```python
from build123d import *

# Parameters (mm, degrees)
F0_R      = 6.35
F1_DEPTH  = 47.625
F3_DEPTH  = 31.75
F4_R      = 23.8125
F4_R_2    = 18.7325
F5_DEPTH  = 20.32
F6_R      = 54.61
F6_R_2    = 6.35
F7_DEPTH  = 14.605
F8_R      = 54.5973
F8_R_2    = 6.35
F9_DEPTH  = 118.491
F10_R     = 54.61
F10_R_2   = 54.5973
F10_R_3   = 6.35
F11_DEPTH = 57.15
F13_DEPTH = 101.6
F15_DEPTH = 25.4
F16_DEPTH = 76.2
F18_DEPTH = 76.2
F20_D     = 12.7
F20_DEPTH = 12.7
F20_TIP   = 3.8154649308
F22_D     = 12.7
F22_2_D   = 12.7
F23_R     = 5.08
F23_2_R   = 5.08


with BuildPart() as f1:
    # F0 (on Top) → F1 (new body)
    with BuildSketch(Plane.XY):
        Circle(F0_R)
    extrude(amount=-F1_DEPTH)

    # F2 (on face) → F3 (cut)
    with BuildSketch(Plane.XY):
        with BuildLine():
            Line((-3.4925, 5.3032955556), (3.4925, 5.3032955556))
            ThreePointArc((3.4925, 5.3032955556), (0, 6.35), (-3.4925, 5.3032955556))
        make_face()
    extrude(amount=-F3_DEPTH, mode=Mode.SUBTRACT)


with BuildPart() as f5:
    # F4 (on face) → F5 (new body)
    with BuildSketch(Plane(origin=(0, 0, -47.625), x_dir=(1, 0, 0), z_dir=(0, 0, -1))):
        Circle(F4_R)
        Circle(F4_R_2, mode=Mode.SUBTRACT)
    extrude(amount=-F5_DEPTH)


with BuildPart() as f7:
    # F6 (on face) → F7 (new body)
    with BuildSketch(Plane(origin=(0, 0, -47.625), x_dir=(1, 0, 0), z_dir=(0, 0, -1))):
        Circle(F6_R)
        Circle(F6_R_2, mode=Mode.SUBTRACT)
    extrude(amount=F7_DEPTH)

    # F8 (on face) → F9 (join)
    with BuildSketch(Plane(origin=(0, 0, -62.23), x_dir=(1, 0, 0), z_dir=(0, 0, -1))):
        Circle(F8_R)
        Circle(F8_R_2, mode=Mode.SUBTRACT)
    extrude(amount=F9_DEPTH)

    # F10 (on face) → F11 (join)
    with BuildSketch(Plane(origin=(0, 0, -180.721), x_dir=(1, 0, 0), z_dir=(0, 0, -1))):
        Circle(F10_R)
        Circle(F10_R_2, mode=Mode.SUBTRACT)
        Circle(F10_R_2)
        Circle(F10_R_3, mode=Mode.SUBTRACT)
    extrude(amount=F11_DEPTH)


with BuildPart() as f13:
    # F12 (on face) → F13 (new body)
    with BuildSketch(Plane.XY.offset(-47.625)):
        with BuildLine():
            Line((-82.55, 31.7245898319), (-44.45, 31.7245898319))
            ThreePointArc((-44.45, 31.7245898319), (-24.9977223891, 48.5527133676), (0, 54.61))
            Line((0, 54.61), (0, 67.31))
            ThreePointArc((0, 67.31), (-26.9947671741, 61.30558596), (-48.8991597124, 44.4245898319))
            Line((-48.8991597124, 44.4245898319), (-82.55, 44.4245898319))
            Line((-82.55, 44.4245898319), (-82.55, 31.7245898319))
        make_face()
        with BuildLine():
            ThreePointArc((0, 54.61), (24.9977223891, 48.5527133676), (44.45, 31.7245898319))
            Line((44.45, 31.7245898319), (82.55, 31.7245898319))
            Line((82.55, 31.7245898319), (82.55, 44.4245898319))
            Line((82.55, 44.4245898319), (48.8991597124, 44.4245898319))
            ThreePointArc((48.8991597124, 44.4245898319), (26.9947671741, 61.30558596), (0, 67.31))
            Line((0, 67.31), (0, 54.61))
        make_face()
    extrude(amount=-F13_DEPTH)

    # F22 (through all)
    with Locations(Plane.XZ.offset(44.4245898319)):
        with Locations((-69.85, -60.325), (-69.85, -98.425), (-69.85, -136.525), (69.85, -60.325), (69.85, -98.425), (69.85, -136.525)):
            Hole(F22_D / 2)

    # F23#2
    f23_2_edges = [f13.edges().sort_by_distance(p)[0] for p in [
        (-48.89916, 44.42459, -98.425),
        (48.89916, 44.42459, -98.425),
    ]]
    fillet(f23_2_edges, radius=F23_2_R)


with BuildPart() as f15:
    # F14 (on face) → F15 (new body)
    with BuildSketch(Plane.XY.offset(-47.625)):
        with BuildLine():
            Line((82.55, -31.7245898319), (44.45, -31.7245898319))
            ThreePointArc((44.45, -31.7245898319), (24.9977223891, -48.5527133676), (0, -54.61))
            Line((0, -54.61), (0, -67.31))
            ThreePointArc((0, -67.31), (26.9947671741, -61.30558596), (48.8991597124, -44.4245898319))
            Line((48.8991597124, -44.4245898319), (82.55, -44.4245898319))
            Line((82.55, -44.4245898319), (82.55, -31.7245898319))
        make_face()
        with BuildLine():
            ThreePointArc((0, -54.61), (-24.9977223891, -48.5527133676), (-44.45, -31.7245898319))
            Line((-44.45, -31.7245898319), (-82.55, -31.7245898319))
            Line((-82.55, -31.7245898319), (-82.55, -44.4245898319))
            Line((-82.55, -44.4245898319), (-48.8991597124, -44.4245898319))
            ThreePointArc((-48.8991597124, -44.4245898319), (-26.9947671741, -61.30558596), (0, -67.31))
            Line((0, -67.31), (0, -54.61))
        make_face()
    extrude(amount=-F15_DEPTH)

    # F16 (add): faces of the model
    f16_faces = [f15.faces().sort_by_distance(p)[0] for p in [
        (80.8610852178, -38.0745898319, -73.025),
        (80.8610852178, -38.0745898319, -73.025),
    ]]
    extrude(f16_faces, amount=F16_DEPTH)

    # F17 (on face) → F18 (join)
    with BuildSketch(Plane(origin=(0, 0, -149.225), x_dir=(1, 0, 0), z_dir=(0, 0, -1))):
        with BuildLine():
            Line((-38.1, 87.6758182624), (-38.1, 54.6558182624))
            ThreePointArc((-38.1, 54.6558182624), (0, 67.31), (38.1, 54.6558182624))
            Line((38.1, 54.6558182624), (38.1, 87.6758182624))
            Line((38.1, 87.6758182624), (12.7, 87.6758182624))
            ThreePointArc((12.7, 87.6758182624), (0, 76.2), (-12.7, 87.6758182624))
            Line((-12.7, 87.6758182624), (-38.1, 87.6758182624))
        make_face()
    extrude(amount=-F18_DEPTH)

    # F20
    with Locations(Plane.XZ.offset(87.6758182624)):
        with Locations((-25.4, -85.725), (25.4, -85.725), (-25.4, -111.125), (25.4, -111.125), (-25.4, -136.525), (25.4, -136.525)):
            Hole(F20_D / 2, depth=F20_DEPTH)
            with Locations((0, 0, -(F20_DEPTH + F20_TIP / 2))):  # 118° drill point
                Cone(0, F20_D / 2, F20_TIP, mode=Mode.SUBTRACT)

    # F22#2 (through all)
    with Locations(Plane.XZ.offset(44.4245898319)):
        with Locations((-69.85, -60.325), (-69.85, -98.425), (-69.85, -136.525), (69.85, -60.325), (69.85, -98.425), (69.85, -136.525)):
            Hole(F22_2_D / 2)

    # F23
    f23_edges = [f15.edges().sort_by_distance(p)[0] for p in [
        (-38.1, -54.655818, -111.125),
        (0, -67.31, -73.025),
        (38.1, -54.655818, -111.125),
        (48.89916, -44.42459, -98.425),
        (-48.89916, -44.42459, -98.425),
    ]]
    fillet(f23_edges, radius=F23_R)


solid = f15.part
```
Geometry: final body of the model. Coordinates: model frame, mm. A direction names the side the tool comes from. Round coordinates to 2 decimals unless told otherwise and drop trailing zeros. Loops run counter-clockwise (first coordinate to the right, second up) from the corner with the lowest first, then second, coordinate; pieces in that order, holes last.
Item 1: Section B-B, the plane x = -69.85. Output: boundary loops of the cut face in (y, z) (3 decimals).
Checked values:
outline: (-44.425, -149.225) - (-31.725, -149.225) - (-31.725, -142.875) - (-44.425, -142.875) - close; (-44.425, -130.175) - (-31.725, -130.175) - (-31.725, -104.775) - (-44.425, -104.775) - close; (-44.425, -92.075) - (-31.725, -92.075) - (-31.725, -66.675) - (-44.425, -66.675) - close; (-44.425, -53.975) - (-31.725, -53.975) - (-31.725, -47.625) - (-44.425, -47.625) - close
Item 2: Reachability of faces 1 (the flat face through (-1, -74, -73.025)), 2 (the flat face through (82.55, -38, -98)) from +Z, -Z, +X, -X, +Y, -Y: full face, straight path, thin tool, end or side. Return the list, or none.
Checked values:
face 1: +Z, -Y
face 2: +Z, -Z, +X, +Y, -Y
Item 3: Mould query, pull axis Z, two halves, no side actions, for faces 3 (the cylindrical face through (38.61, -54.92, -108.02)), 4 (the cylindrical face through (26.777, -81.237, -117.324)), 5 (the flat face through (-1, -60, -149.225)). Classes: released by +Z, released by -Z, zero draft, split by the parting line, or undercut.
Checked values:
face 3: zero draft
face 4: undercut
face 5: released by -Z
Item 4: Line query: L1, parallel to Z at x = 25, y = -80 (3 decimals); L2, parallel to Z at x = 71, y = -38.5 (3 decimals); L3, parallel to X at y = -81, z = -116. Output: solid intervals per line, ascending.
Checked values:
L1: z = -149.225 to -142.862, -130.188 to -117.462, -104.788 to -92.062, -79.388 to -73.025
L2: z = -149.225 to -142.77, -130.28 to -104.67, -92.18 to -66.57, -54.08 to -47.625
L3: x = -38.1 to -29.47, -21.33 to -9.98, 9.98 to 21.33, 29.47 to 38.1
Item 5: Section D-D, the plane y = -41. Output: boundary loops of the cut face in (x, z) (3 decimals).
Checked values:
outline: (-82.55, -149.225) - (-36.073, -149.225) - (-36.073, -47.625) - (-82.55, -47.625) - close; (36.073, -149.225) - (82.55, -149.225) - (82.55, -47.625) - (36.073, -47.625) - close; hole circle Ø12.7 at (-69.85, -136.525); hole circle Ø12.7 at (-69.85, -98.425); hole circle Ø12.7 at (-69.85, -60.325); hole circle Ø12.7 at (69.85, -136.525); hole circle Ø12.7 at (69.85, -98.425); hole circle Ø12.7 at (69.85, -60.325)
Item 6: Contact query for flat-ended pins moving along their axis: P1, Ø15.5, axis at x = 69, z = -88.5, coming from the -Y side; P2, Ø10, axis at x = 25.4, z = -136.525, coming from the +Y side; P3, Ø8, axis at x = 37, z = -97, coming from the +Y side; P4, Ø10, axis at x = 69.85, z = -60.325, coming from the +Y side. Output: stop coordinate, or through.
Checked values:
P1: stops at y = -44.42
P2: stops at y = -45.37
P3: stops at y = -36.07
P4: passes through
Item 7: Section C-C, the plane z = -58.5. Output: boundary loops of the cut face in (x, y).
Checked values:
outline: (-82.55, -44.42) - (-75.93, -44.42) - (-75.93, -31.72) - (-82.55, -31.72) - close; (-63.77, -44.42) - (-51.22, -44.42) arc R5.08 cw to (-47.44, -46.12) arc R63.68 ccw to (47.44, -46.12) arc R5.08 cw to (51.22, -44.42) - (63.77, -44.42) - (63.77, -31.72) - (44.45, -31.72) arc R54.61 cw to (-44.45, -31.72) - (-63.77, -31.72) - close; (75.93, -44.42) - (82.55, -44.42) - (82.55, -31.72) - (75.93, -31.72) - close
Item 8: Section A-A, the plane y = -82. Output: boundary loops of the cut face in (x, z) (3 decimals), plus the area to 3 significant figures.
Checked values:
outline: (-38.1, -149.225) - (-10.698, -149.225) - (-10.698, -73.025) - (-38.1, -73.025) - close; (10.698, -149.225) - (38.1, -149.225) - (38.1, -73.025) - (10.698, -73.025) - close; hole circle Ø12.7 at (-25.4, -136.525); hole circle Ø12.7 at (-25.4, -111.125); hole circle Ø12.7 at (-25.4, -85.725); hole circle Ø12.7 at (25.4, -136.525); hole circle Ø12.7 at (25.4, -111.125); hole circle Ø12.7 at (25.4, -85.725)
area: 3,420 mm2
